from build123d import *

# Parameters (mm, degrees)
SKETCH1_W           = 54.3999928
SKETCH1_H           = 34.7000068
BOSS_EXTRUDE1_DEPTH = 3.999992
SKETCH2_R           = 3.125000785
CUT_EXTRUDE1_DEPTH  = 2.999994
SKETCH7_R           = 1.7499965
CUT_EXTRUDE5_DEPTH  = 33.401579995
SKETCH8_R           = 0.621776252
SKETCH8_R_2         = 0.622309086
CUT_EXTRUDE6_DEPTH  = 33.509419529
CUT_EXTRUDE7_DEPTH  = 2.999994


with BuildPart() as part:
    # Sketch1 → Boss-Extrude1 (new body)
    with BuildSketch(Plane(origin=(0, 0, 0), x_dir=(1, 0, 0), z_dir=(0, 1, 0))):
        Rectangle(SKETCH1_W, SKETCH1_H)
    extrude(amount=BOSS_EXTRUDE1_DEPTH)

    # Sketch2 → Cut-Extrude1 (cut)
    with BuildSketch(Plane(origin=(0, 3.999992, 0), x_dir=(1, 0, 0), z_dir=(0, 1, 0))):
        with Locations(Location((-19.999997415, 0, 0), (0, 0, 270))):
            Circle(SKETCH2_R)
        with Locations(Location((19.999997415, 0, 0), (0, 0, 90))):
            Circle(SKETCH2_R)
    extrude(amount=-CUT_EXTRUDE1_DEPTH, mode=Mode.SUBTRACT)

    # Sketch7 → Cut-Extrude5 (cut, through all)
    with BuildSketch(Plane(origin=(0, 0.999998, 0), x_dir=(1, 0, 0), z_dir=(0, 1, 0))):
        with Locations(Location((-19.999997415, 0, 0), (0, 0, 270))):
            Circle(SKETCH7_R)
        with Locations(Location((19.999997415, 0, 0), (0, 0, 90))):
            Circle(SKETCH7_R)
    extrude(amount=-CUT_EXTRUDE5_DEPTH, mode=Mode.SUBTRACT)

    # Sketch8 → Cut-Extrude6 (cut, through all)
    with BuildSketch(Plane(origin=(0, 3.999992, 0), x_dir=(1, 0, 0), z_dir=(0, 1, 0))):
        with Locations(Location((-13.914038205, -0.000532834, 0), (0, 0, 270))):
            Circle(SKETCH8_R)
        with Locations(Location((-11.925423769, 0, 0), (0, 0, 270))):
            Circle(SKETCH8_R_2)
        with Locations(Location((-9.936809177, -0.000532834, 0), (0, 0, 270))):
            Circle(SKETCH8_R)
        with Locations(Location((-7.948194741, 0, 0), (0, 0, 270))):
            Circle(SKETCH8_R_2)
        with Locations(Location((-5.959580149, -0.000532834, 0), (0, 0, 270))):
            Circle(SKETCH8_R)
        with BuildLine():
            ThreePointArc((3.60507443, 0.503380738), (4.593274799, 0), (3.60507443, -0.503380738))
            ThreePointArc((3.60507443, -0.503380738), (0, -3.6400486), (-3.60507443, -0.503380738))
            ThreePointArc((-3.60507443, -0.503380738), (-4.593274799, 0), (-3.60507443, 0.503380738))
            ThreePointArc((-3.60507443, 0.503380738), (0, 3.6400486), (3.60507443, 0.503380738))
        make_face()
        with Locations(Location((5.959580149, -0.000532834, 0), (0, 0, 270))):
            Circle(SKETCH8_R)
        with Locations(Location((9.936809177, -0.000532834, 0), (0, 0, 270))):
            Circle(SKETCH8_R)
        with Locations(Location((7.948194741, 0, 0), (0, 0, 270))):
            Circle(SKETCH8_R_2)
        with Locations(Location((11.925423769, 0, 0), (0, 0, 270))):
            Circle(SKETCH8_R_2)
        with Locations(Location((13.914038205, -0.000532834, 0), (0, 0, 270))):
            Circle(SKETCH8_R)
    extrude(amount=-CUT_EXTRUDE6_DEPTH, mode=Mode.SUBTRACT)

    # Sketch9 → Cut-Extrude7 (cut)
    with BuildSketch(Plane(origin=(0, 3.999992, 0), x_dir=(1, 0, 0), z_dir=(0, 1, 0))):
        with BuildLine():
            Line((-14.2410688, 2.2370542), (-0.4017772, 3.7338))
            ThreePointArc((-0.4017772, 3.7338), (0, 3.755463322), (0.4017772, 3.7338))
            Line((0.4017772, 3.7338), (14.2410688, 2.2370542))
            ThreePointArc((14.2410688, 2.2370542), (16.250002136, 0), (14.2410688, -2.2370542))
            Line((14.2410688, -2.2370542), (0.4017772, -3.7338))
            ThreePointArc((0.4017772, -3.7338), (0, -3.755463322), (-0.4017772, -3.7338))
            Line((-0.4017772, -3.7338), (-14.2410688, -2.2370542))
            ThreePointArc((-14.2410688, -2.2370542), (-16.250002136, 0), (-14.2410688, 2.2370542))
        make_face()
    extrude(amount=-CUT_EXTRUDE7_DEPTH, mode=Mode.SUBTRACT)


solid = part.part
Geometry check sheet. Reference: the model listing, model coordinates, mm. A direction names the side the tool comes from. Round coordinates to 2 decimals unless told otherwise and drop trailing zeros. Loops run counter-clockwise (first coordinate to the right, second up) from the corner with the lowest first, then second, coordinate; pieces in that order, holes last.
Item 1: Access from +Z, -Z, +X, -X, +Y, -Y to the whole of each face (thin tool, end or side, straight path). Record for faces 4 (the flat face through (21.35, 1, -1.35)), 5 (the cylindrical face through (-9.32, 0.51, -0.08)).
Item 2: Thickness scan on line 1 (Z direction, x = 20, y = 1.2) (3 decimals); line 2 (X direction, y = 1.95, z = 2); line 3 (X direction, y = 1.4, z = 1). Record the ranges inside material, lowest first.
Item 3: Gauge pin test, flat ends, axial feed: pin 1 (1 mm diameter, centred on x = 7.95, z = 0, fed in from -Y); pin 2 (1.9 mm diameter, centred on x = -20, z = 1.5, fed in from +Y). Record the tip position at first contact, or that the pin passes through.
Item 4: Mould release check, pull along Z, two halves, no side actions. Record for faces 1 (the flat face through (7.418, 2.521, 2.975)), 2 (the flat face through (0, 2, -17.35)), 3 (the flat face through (27.2, 2, 0)): pulls with the +Z half, pulls with the -Z half, needs draft (parallel to the pull), parting line crosses it, or undercut.
Item 5: Cross-section at A-A on y = 3.05. Record the boundary of the cut face in (x, z) (3 decimals).
Item 6: Cross-section at B-B on x = -2.5. Record the boundary of the cut face in (y, z), then the cut area to 3 significant figures.
Answer sheet:
1. face 4: +Y
1. face 5: +Y, -Y
2. line 1: z = -17.35 to -3.125, 3.125 to 17.35
2. line 2: x = -27.2 to -22.4, -17.6 to -15.03, 15.03 to 17.6, 22.4 to 27.2
2. line 3: x = -27.2 to -22.96, -17.04 to -16.02, 16.02 to 17.04, 22.96 to 27.2
3. pin 1: passes through
3. pin 2: stops at y = 1
4. face 1: undercut
4. face 2: pulls with the -Z half
4. face 3: needs draft
5. outline: (-27.2, -17.35) - (27.2, -17.35) - (27.2, 17.35) - (-27.2, 17.35) - close; hole circle Ø6.25 at (-20, 0); hole (-14.241, -2.237) - (-0.402, -3.734) arc R3.737 ccw to (0.402, -3.734) - (14.241, -2.237) arc R2.25 ccw to (14.241, 2.237) - (0.402, 3.734) arc R3.737 ccw to (-0.402, 3.734) - (-14.241, 2.237) arc R2.25 ccw to start; hole circle Ø6.25 at (20, 0)
6. outline: (0, -17.35) - (4, -17.35) - (4, -3.51) - (1, -3.51) - (1, -2.65) - (0, -2.65) - close; (0, 2.65) - (1, 2.65) - (1, 3.51) - (4, 3.51) - (4, 17.35) - (0, 17.35) - close
6. area: 112 mm2
